```python
from build123d import *

# Parameters (mm, degrees)
SKETCH1_R           = 15
BOSS_EXTRUDE1_DEPTH = 40
BOSS_EXTRUDE2_START = -20
SKETCH2_R           = 15
BOSS_EXTRUDE2_DEPTH = 20


with BuildPart() as part:
    # Sketch1 → Boss-Extrude1 (new body)
    with BuildSketch(Plane.XY):
        Circle(SKETCH1_R)
        with BuildLine():
            Line((2.010289907, 10), (2.010289907, 5.970656119))
            ThreePointArc((2.010289907, 5.970656119), (5.116386733, 3.675947061), (6.3, 0))
            ThreePointArc((6.3, 0), (-3.680353244, -5.113218165), (-2, 5.974110812))
            Line((-2, 5.974110812), (-2, 10))
            Line((-2, 10), (2.010289907, 10))
        make_face(mode=Mode.SUBTRACT)
    extrude(amount=BOSS_EXTRUDE1_DEPTH)

    # Sketch2 → Boss-Extrude2 (add)
    with BuildSketch(Plane.XY.offset(40).offset(BOSS_EXTRUDE2_START)):
        Circle(SKETCH2_R)
    extrude(amount=BOSS_EXTRUDE2_DEPTH)


solid = part.part
```
For this review, take the finished solid that the model builds, in its own axes (mm). A direction names the side the tool comes from. Round coordinates to 2 decimals unless told otherwise and drop trailing zeros. Write each loop counter-clockwise with the first axis right and the second up, starting at its lowest first coordinate (ties: lowest second). Pieces come first, ordered by that corner, then holes. Notation, with made-up numbers: (-19.5, 8) - (30.5, 8) arc R23 cw to (30.5, 16) - close; hole circle Ø1 at (42.25, -16). An arc over 180 degrees is marked (long way). Answer as CSV lines item,"result". Start each with the question number.
(1) Add section A-A, the plane y = 9. State the section outline as (x, z) points.
(2) Add section C-C, the plane z = 9. State the section outline as (x, y) points.
(3) For pin 1 (4.5 mm diameter, centred on y = 7, z = 11, fed in from -X); pin 2 (8 mm diameter, centred on x = -9, z = 31, fed in from +Y); pin 3 (2 mm diameter, centred on y = 8.5, z = 5.5, fed in from +X), all flat-tipped, find the tip position at first contact; note any pin that passes through.
(4) Mouldability with a two-part tool opening along Y and no side actions: class faces 3 (the flat face through (0, 0, 40)), 4 (the cylindrical face through (-14.985, 0.66, 19.72)), 5 (the flat face through (0, 0, 20)) as +Y half, -Y half, draft (parallel to the pull), parting line (faces both ways), or undercut.
(5) Add section B-B, the plane x = 0. State the section outline as (y, z) points.
(6) Add section D-D, the plane y = -7.25. State the section outline as (x, z) points.
(7) For line 1 (Y direction, x = 0, z = 14); line 2 (X direction, y = -0.5, z = 33); line 3 (Z direction, x = -1.5, y = -4.75), list the stretches that pass through material, from the lowest coordinate up.
(8) Machinability: for faces 1 (the flat face through (-0.2, -6.5, 0)), 2 (the flat face through (-2, 8, 10)), which of the approach directions +Z, -Z, +X, -X, +Y, -Y give a long, thin tool a straight path to every point of the face, cutting with its end or side? Answer none if there is none.
From the geometry:
1,outline,"(-12, 0) - (-2, 0) - (-2, 20) - (2.01, 20) - (2.01, 0) - (12, 0) - (12, 40) - (-12, 40) - close"
2,outline,"circle Ø30 at (0, 0); hole (-2, 5.97) arc R6.3 ccw (long way) to (2.01, 5.97) - (2.01, 10) - (-2, 10) - close"
3,pin 1,"stops at x = -14.23"
3,pin 2,"stops at y = 14.14"
3,pin 3,"stops at x = 12.99"
4,face 3,"draft"
4,face 4,"parting line"
4,face 5,"undercut"
5,outline,"(-15, 0) - (-6.3, 0) - (-6.3, 20) - (10, 20) - (10, 0) - (15, 0) - (15, 40) - (-15, 40) - close"
6,outline,"(-13.13, 0) - (13.13, 0) - (13.13, 40) - (-13.13, 40) - close"
7,line 1,"y = -15 to -6.3, 10 to 15"
7,line 2,"x = -14.99 to 14.99"
7,line 3,"z = 20 to 40"
8,face 1,"-Z, +X, -X, +Y, -Y"
8,face 2,"-Z"
